Design review of the part built by this model. Coordinates are the model's own, in mm. A direction names the side the tool comes from. Coordinates: 2 decimals unless noted, no trailing zeros. Write each loop counter-clockwise with the first axis right and the second up, starting at its lowest first coordinate (ties: lowest second). Pieces come first, ordered by that corner, then holes. Notation, with made-up numbers: M -23.5,85.25 L 8.5,85.25 A27 cw 8.5,116.25 Z; hole C 49.25,-20.5 d10. An arc over 180 degrees is marked long. Write item = value, one per line.
```python
from build123d import *

# Parameters (mm, degrees)
F0_W     = 6
F0_H     = 3.9
F0_W_2   = 5.6
F0_H_2   = 3
F1_DEPTH = 10
F3_DEPTH = 1
F4_SIZE  = 0.8
F5_W     = 0.6
F5_H     = 8
F6_DEPTH = 1
F7_SIZE  = 0.8
F8_W     = 0.6
F8_H     = 8
F9_DEPTH = 1
F10_SIZE = 0.8


with BuildPart() as f1:
    # F0 (on Top) → F1 (new body)
    with BuildSketch(Plane.XY):
        Rectangle(F0_W, F0_H)
        with Locations((0, -0.15)):
            Rectangle(F0_W_2, F0_H_2, mode=Mode.SUBTRACT)
    extrude(amount=F1_DEPTH)

    # F2 (on face) → F3 (join)
    with BuildSketch(Plane.XZ.offset(1.95)):
        Polygon((1, 9), (-1, 9), (-1, 3), (-2, 3), (-1, 1.5), (0, 1.5), (1, 1.5), (2, 3), (1, 3), align=None)
    extrude(amount=F3_DEPTH)

    # F4
    f4_edges = [f1.edges().sort_by_distance(p)[0] for p in [
        (0, -2.95, 1.5),
    ]]
    chamfer(f4_edges, length=F4_SIZE)

    # F5 (on face) → F6 (join)
    with BuildSketch(Plane.YZ.offset(3)):
        with Locations((-1.65, 6)):
            Rectangle(F5_W, F5_H)
    extrude(amount=F6_DEPTH)

    # F7
    f7_edges = [f1.edges().sort_by_distance(p)[0] for p in [
        (4, -1.65, 2),
    ]]
    chamfer(f7_edges, length=F7_SIZE)

    # F8 (on face) → F9 (join)
    with BuildSketch(Plane(origin=(-3, 0, 0), x_dir=(0, -1, 0), z_dir=(-1, 0, 0))):
        with Locations((1.65, 6)):
            Rectangle(F8_W, F8_H)
    extrude(amount=F9_DEPTH)

    # F10
    f10_edges = [f1.edges().sort_by_distance(p)[0] for p in [
        (-4, -1.65, 2),
    ]]
    chamfer(f10_edges, length=F10_SIZE)


solid = f1.part
```
Q1. For P1, Ø0.8, axis at y = -2.5, z = 7, coming from the -X side; P2, Ø2, axis at x = 0, y = -1.5, coming from the +Z side; P3, Ø2, axis at y = 0.5, z = 3.5, coming from the +X side; P4, Ø1.5, axis at x = -0.5, y = -0.5, coming from the -Z side, all flat-tipped, find the tip position at first contact; note any pin that passes through.
Check result:
P1 = -1
P2 = 10
P3 = 3
P4 = through
Q2. Consider section A-A, the plane y = 0.6. State the section outline as (x, z) points, and give its area (3 significant figures).
Check result:
outline = M -3,0 L -2.8,0 L -2.8,10 L -3,10 Z; M 2.8,0 L 3,0 L 3,10 L 2.8,10 Z
area = 4.00 mm²
Q3. Wall thickness on line 1 (Y direction, x = 0.75, z = 6.25); line 2 (Y direction, x = 1.5, z = 1.25); line 3 (X direction, y = -0.6, z = 7.5): over which ranges is each line inside the solid? List them lowest first.
Check result:
line_1 = -2.95 to -1.65, 1.35 to 1.95
line_2 = -1.95 to -1.65, 1.35 to 1.95
line_3 = -3 to -2.8, 2.8 to 3
Q4. Consider section C-C, the plane z = 3.25. State the section outline as (x, y) points.
Check result:
outline = M -4,-1.95 L -1,-1.95 L -1,-2.95 L 1,-2.95 L 1,-1.95 L 4,-1.95 L 4,-1.35 L 3,-1.35 L 3,1.95 L -3,1.95 L -3,-1.35 L -4,-1.35 Z; hole M -2.8,-1.65 L 2.8,-1.65 L 2.8,1.35 L -2.8,1.35 Z
Q5. Consider section B-B, the plane x = 0.25. State the section outline as (y, z) points, and give its area (3 significant figures).
Check result:
outline = M -2.95,2.3 L -2.15,1.5 L -1.95,1.5 L -1.95,0 L -1.65,0 L -1.65,10 L -1.95,10 L -1.95,9 L -2.95,9 Z; M 1.35,0 L 1.95,0 L 1.95,10 L 1.35,10 Z
area = 16.2 mm²
Q6. Machinability: for faces 1 (the flat face through (-1.6, -2.3, 2.4)), 2 (the flat face through (-1.5, -2.4, 3)), 3 (the flat face through (1, -2.4, 6)), 4 (the flat face through (0, 1.35, 5)), 5 (the flat face through (1.6, -2.3, 2.4)), which of the approach directions +Z, -Z, +X, -X, +Y, -Y give a long, thin tool a straight path to every point of the face, cutting with its end or side? Answer none if there is none.
Check result:
face_1 = -Z, -X, -Y
face_2 = +Z, -X, -Y
face_3 = +Z, +X, -Y
face_4 = +Z, -Z
face_5 = -Z, +X, -Y
Q7. Consider section D-D, the plane x = -2.25. State the section outline as (y, z) points.
Check result:
outline = M -1.95,0 L -1.65,0 L -1.65,10 L -1.95,10 Z; M 1.35,0 L 1.95,0 L 1.95,10 L 1.35,10 Z
